```python
from build123d import *

# Parameters (mm, degrees)
SKETCH_W     = 120
SKETCH_H     = 40
PAD_DEPTH    = 10
SKETCH001_W  = 120
SKETCH001_H  = 10
PAD001_DEPTH = 20
PAD002_DEPTH = 24.6


with BuildPart() as part:
    # Sketch → Pad (new body)
    with BuildSketch(Plane.XY):
        with Locations((-60, 20)):
            Rectangle(SKETCH_W, SKETCH_H)
    extrude(amount=PAD_DEPTH)

    # Sketch001 (on Face6 of Pad) → Pad001 (join)
    with BuildSketch(Plane.XY.offset(10)):
        with Locations((-60, 15)):
            Rectangle(SKETCH001_W, SKETCH001_H)
    extrude(amount=PAD001_DEPTH)

    # Sketch002 (on Face8 of Pad001) → Pad002 (join)
    with BuildSketch(Plane.YZ):
        Polygon((15.4, 30), (15.4, 6.4), (36.6, 6.4), (36.6, 10), (20, 10), (20, 30), align=None)
    extrude(amount=PAD002_DEPTH)


solid = part.part
```
Work out the finished part from the listing and answer in its coordinate system (mm). A direction names the side the tool comes from. Give positions to 0.01 mm unless a question says otherwise; leave off trailing zeros. Loops run counter-clockwise (first coordinate to the right, second up) from the corner with the lowest first, then second, coordinate; pieces in that order, holes last. Notation, with made-up numbers: (-25.5, 79) -> (21.5, 79) arc R14 ccw to (21.5, 87) -> close; hole circle Ø7 at (-31.5, 84). An arc over 180 degrees is marked (long way). Put each result on its own line as item: value. Start each with the question number.
Item 1: The part is cut by section A-A (x = -27.5). Give the vertices of the cut face in (y, z).
Item 2: The part is cut by section D-D (z = 2.25). Give the vertices of the cut face in (x, y).
Item 3: Which of the six approach directions +Z, -Z, +X, -X, +Y, -Y give full straight-line access (tool end or side, diameter ignored) to faces 1 (the face through (-61, 10, 20)), 2 (the face through (12, 36.6, 8)), 3 (the face through (12, 26, 6.4))?
Item 4: Find the intervals of material crossed by L1, parallel to Z at x = -103.5, y = 22; L2, parallel to Y at x = -99, z = 14.5; L3, parallel to X at y = 21, z = 5.5, in increasing order. Write a range as [from, to].
Item 5: The part is cut by section C-C (z = 22). Give the vertices of the cut face in (x, y).
Item 6: Each of these flat-tipped pins is pushed along its axis until it touches: P1, Ø11, axis at x = -58, y = 6, coming from the +Z side; P2, Ø6.5, axis at x = 17.5, y = 29.5, coming from the -Z side; P3, Ø4, axis at x = -69.5, y = 6, coming from the +Z side; P4, Ø10, axis at x = -39.5, z = 20, coming from the -Y side. Where does it stop, or does it pass through?
Item 7: The part is cut by section B-B (y = 31). Give the vertices of the cut face in (x, z).
Answers below:
1. outline: (0, 0) -> (40, 0) -> (40, 10) -> (20, 10) -> (20, 30) -> (10, 30) -> (10, 10) -> (0, 10) -> close
2. outline: (-120, 0) -> (0, 0) -> (0, 40) -> (-120, 40) -> close
3. face 1: +Z, +X, -X, -Y
3. face 2: +Z, -Z, +X, +Y
3. face 3: -Z, +X, +Y, -Y
4. L1: [0, 10]
4. L2: [10, 20]
4. L3: [-120, 0]
5. outline: (-120, 10) -> (0, 10) -> (0, 15.4) -> (24.6, 15.4) -> (24.6, 20) -> (-120, 20) -> close
6. P1: z = 30
6. P2: z = 6.4
6. P3: z = 10
6. P4: y = 10
7. outline: (-120, 0) -> (0, 0) -> (0, 6.4) -> (24.6, 6.4) -> (24.6, 10) -> (-120, 10) -> close
